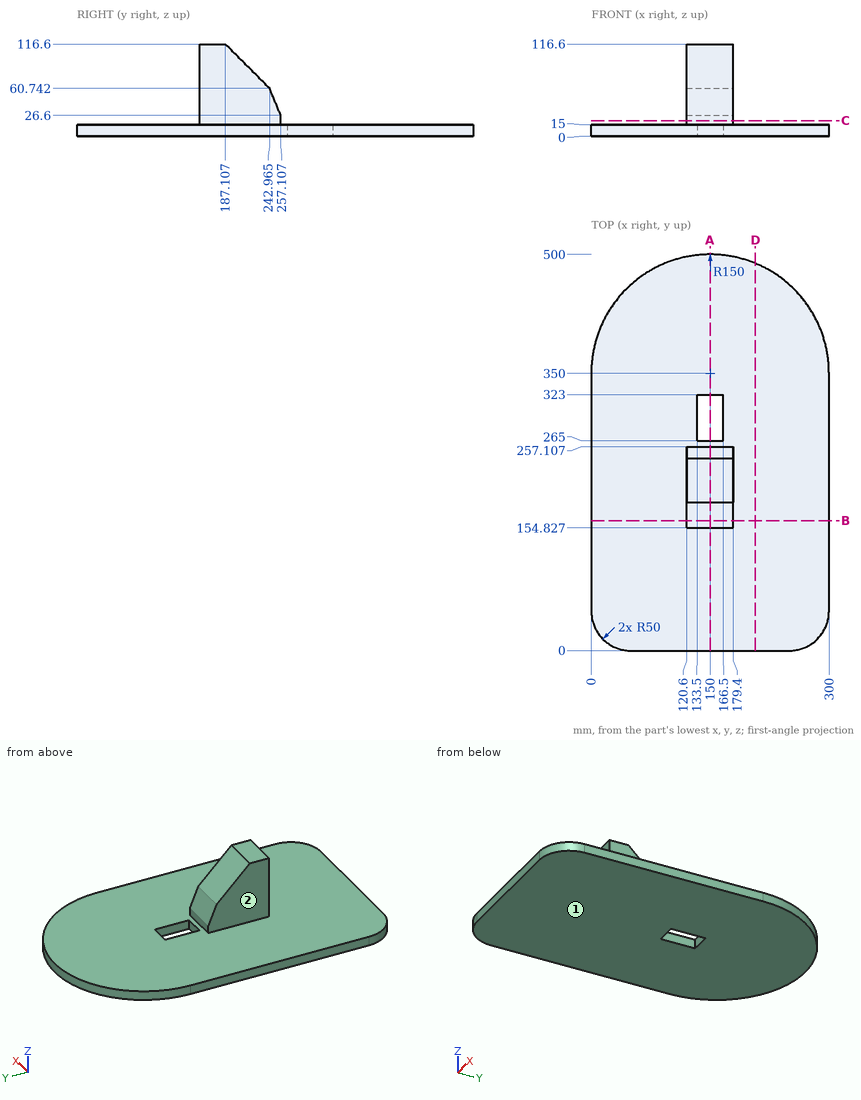
Verification items for this drawing (mm, ordinates from the low corner). A direction names the side the tool comes from. Give positions to 0.01 mm unless a question says otherwise; leave off trailing zeros. Write each loop counter-clockwise with the first axis right and the second up, starting at its lowest first coordinate (ties: lowest second). Pieces come first, ordered by that corner, then holes. Notation, with made-up numbers: (19.25, -3) -> (25.25, -3) arc R10 ccw to (25.25, 15) -> close; hole circle Ø1 at (57.5, 28). An arc over 180 degrees is marked (long way). Use CSV: the item, a comma, the result in double quotes. Start each with the question number.
Q1. Cross-section at B-B on y = 164. Enter the section's corners in (x, z), and give its area (3 significant figures).
Q2. Scan lines: line 1 along Z through (x, y) = (270.5, 197.5); line 2 along Y through (x, z) = (122.5, 23); line 3 along X through (y, z) = (230, 66). Record each from-to range of solid material in increasing order.
Q3. Cross-section at A-A on x = 150. Enter the section's corners in (y, z) (3 decimals).
Q4. Cross-section at C-C on z = 20. Enter the section's corners in (x, y).
Q5. Cross-section at D-D on x = 207. Enter the section's corners in (y, z).
Q6. Tool access check on the marked faces 1 and 2. Record the directions out of +Z, -Z, +X, -X, +Y, -Y that give a thin tool (end or side, any length) a straight path to the whole face; none if there is none.
Q7. Depth check by flat-ended pin: P1, Ø4.5, axis at y = 287.5, z = 8.5, coming from the -X side; P2, Ø3, axis at x = 224.5, y = 332.5, coming from the +Z side; P3, Ø6, axis at y = 173, z = 35.5, coming from the -X side. Enter the tip coordinate at first touch or a pass-through.
Working result:
1,outline,"(0, 0) -> (300, 0) -> (300, 15) -> (179.4, 15) -> (179.4, 116.6) -> (120.6, 116.6) -> (120.6, 15) -> (0, 15) -> close"
1,area,"10,500 mm^2"
2,line 1,"z = 0 to 15"
2,line 2,"y = 154.83 to 257.11"
2,line 3,"x = 120.6 to 179.4"
3,outline,"(0, 0) -> (265, 0) -> (265, 15) -> (257.107, 15) -> (257.107, 26.6) -> (242.965, 60.742) -> (187.107, 116.6) -> (154.827, 116.6) -> (154.827, 15) -> (0, 15) -> close; (323, 0) -> (500, 0) -> (500, 15) -> (323, 15) -> close"
4,outline,"(120.6, 154.83) -> (179.4, 154.83) -> (179.4, 257.11) -> (120.6, 257.11) -> close"
5,outline,"(0, 0) -> (488.75, 0) -> (488.75, 15) -> (0, 15) -> close"
6,face 1,"-Z, +X, -X, +Y, -Y"
6,face 2,"+Z, -X, +Y, -Y"
7,P1,"stops at x = 0"
7,P2,"stops at z = 15"
7,P3,"stops at x = 120.6"
